```python
from build123d import *

# Parameters (mm, degrees)
SKETCH2_W                                      = 144
SKETCH2_H                                      = 20
BOSS_EXTRUDE1_DEPTH                            = 6
CSK_FOR_M2_FLAT_HEAD_MACHINE_SCREW2_AT_2_COUNT = 2
CSK_FOR_M2_FLAT_HEAD_MACHINE_SCREW2_AT_2_PITCH = 70


with BuildPart() as part:
    # Sketch2 → Boss-Extrude1 (new body)
    with BuildSketch(Plane(origin=(0, 0, 0), x_dir=(1, 0, 0), z_dir=(0, 1, 0))):
        with Locations((72, 10)):
            Rectangle(SKETCH2_W, SKETCH2_H)
    extrude(amount=BOSS_EXTRUDE1_DEPTH)

    # Sketch6 → CSK for M2 Flat Head Machine Screw2 (revolve, cut)
    with BuildSketch(Plane(origin=(38, 6, -10), x_dir=(0, 0, 1), z_dir=(1, 0, 0))):
        Polygon((0, 0), (0, 6), (3, 6), (3, 1.207106781), (3.5, 0), align=None)
    csk_for_m2_flat_head_machine_screw2 = revolve(axis=Axis((38, 12.35, -10), (0, -1, 0)), mode=Mode.SUBTRACT)

    # CSK for M2 Flat Head Machine Screw2 at 2: CSK for M2 Flat Head Machine Screw2 ×2
    with Locations(*[(i * CSK_FOR_M2_FLAT_HEAD_MACHINE_SCREW2_AT_2_PITCH, 0, 0) for i in range(1, CSK_FOR_M2_FLAT_HEAD_MACHINE_SCREW2_AT_2_COUNT)]):
        add(csk_for_m2_flat_head_machine_screw2, mode=Mode.SUBTRACT)


solid = part.part
```
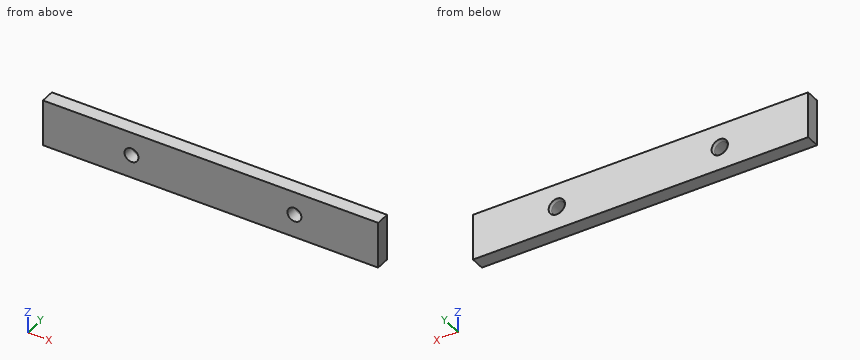
Source: CAD feature listing. Evaluate the final solid. Frame: model axes, mm. Give positions to 0.01 mm unless a question says otherwise; leave off trailing zeros. Loops run counter-clockwise (first coordinate to the right, second up) from the corner with the lowest first, then second, coordinate; pieces in that order, holes last. Notation, with made-up numbers: (-24.5, -19) - (-0.5, -19) arc R20 cw to (-0.5, -14) - close; hole circle Ø9 at (65.25, 74). An arc over 180 degrees is marked (long way). Use CSV: the item, a comma, the result in double quotes. Start each with the question number.
1. Ray query, L1, parallel to X at y = 3.55, z = -10; L2, parallel to Z at x = 38, y = 3.45; L3, parallel to X at y = 2.1, z = -11. Return the intervals inside material, ascending.
2. Section A-A (x = 108). Output: boundary loops of the cut face in (y, z).
3. Section C-C (y = 3.7). Output: boundary loops of the cut face in (x, z), then the cut area to 3 significant figures.
4. Section B-B (z = -10). Output: boundary loops of the cut face in (x, y), then the cut area to 3 significant figures.
Response:
1,L1,"0 to 35, 41 to 105, 111 to 144"
1,L2,"-20 to -13, -7 to 0"
1,L3,"0 to 35.17, 40.83 to 105.17, 110.83 to 144"
2,outline,"(0, -20) - (6, -20) - (6, -13.5) - (4.79, -13) - (0, -13) - close; (0, -7) - (4.79, -7) - (6, -6.5) - (6, 0) - (0, 0) - close"
3,outline,"(0, -20) - (144, -20) - (144, 0) - (0, 0) - close; hole circle Ø6 at (38, -10); hole circle Ø6 at (108, -10)"
3,area,"2,820 mm²"
4,outline,"(0, 0) - (35, 0) - (35, 4.79) - (34.5, 6) - (0, 6) - close; (41, 0) - (105, 0) - (105, 4.79) - (104.5, 6) - (41.5, 6) - (41, 4.79) - close; (111, 0) - (144, 0) - (144, 6) - (111.5, 6) - (111, 4.79) - close"
4,area,"791 mm²"
